Check sheet for the drawn part. Datum: minimum x, y, z corner. Units: mm. Give positions to 0.01 mm unless a question says otherwise; leave off trailing zeros. Write each loop counter-clockwise with the first axis right and the second up, starting at its lowest first coordinate (ties: lowest second). Pieces come first, ordered by that corner, then holes. Notation, with made-up numbers: (26, 60) - (64, 60) arc R25 ccw to (64, 86) - close; hole circle Ø9 at (-27, 9.5). An arc over 180 degrees is marked (long way). Return JSON: item names as keys, results as strings. Group by question number.
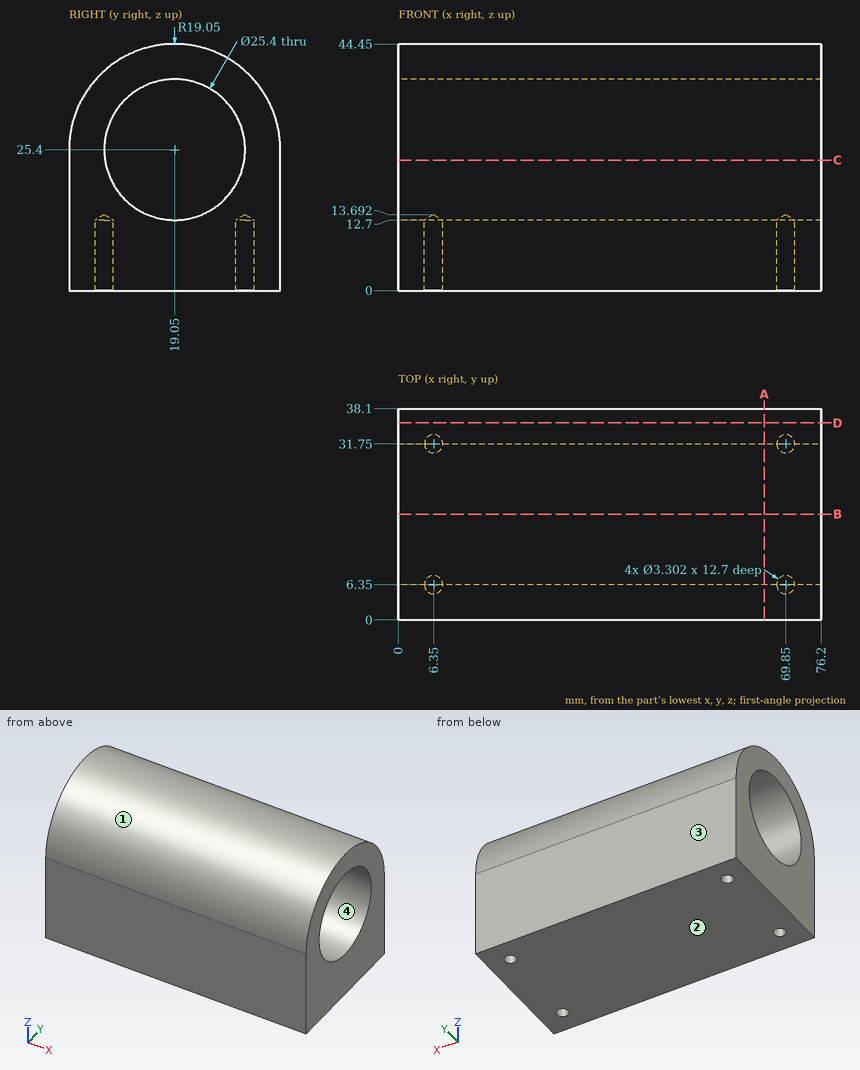
Item 1: Depth check by flat-ended pin: pin 1 (2 mm diameter, centred on x = 6.35, y = 6.35, fed in from +Z); pin 2 (3 mm diameter, centred on x = 6.35, y = 31.75, fed in from -Z); pin 3 (2.5 mm diameter, centred on x = 69.85, y = 6.35, fed in from -Z). Enter the tip coordinate at first touch or a pass-through.
Item 2: Section check B-B on y = 19.05. Record the cut outline in (x, z).
Item 3: Section check C-C on z = 23.5. Record the cut outline in (x, y).
Item 4: Section check A-A on x = 66. Record the cut outline in (y, z).
Item 5: Material ranges on line 1 along Y through (x, z) = (69.85, 7); line 2 along X through (y, z) = (6, 7); line 3 along X through (y, z) = (31, 6), recorded low to high. Write a range as from..to.
Item 6: Mould release check, pull along Z, two halves, no side actions. Record for the marked faces 1, 2, 3 and 4: +Z half, -Z half, draft (parallel to the pull), parting line (faces both ways), or undercut.
Item 7: Section check D-D on y = 35.5. Record the cut outline in (x, z), plus the area to 3 significant figures.
Reply:
{
 "1": {"pin 1": "z = 40.43", "pin 2": "z = 12.79", "pin 3": "z = 12.94"},
 "2": {"outline": "(0, 0) - (76.2, 0) - (76.2, 12.7) - (0, 12.7) - close; (0, 38.1) - (76.2, 38.1) - (76.2, 44.45) - (0, 44.45) - close"},
 "3": {"outline": "(0, 0) - (76.2, 0) - (76.2, 6.49) - (0, 6.49) - close; (0, 31.61) - (76.2, 31.61) - (76.2, 38.1) - (0, 38.1) - close"},
 "4": {"outline": "(0, 0) - (38.1, 0) - (38.1, 25.4) arc R19.05 ccw to (0, 25.4) - close; hole circle Ø25.4 at (19.05, 25.4)"},
 "5": {"line 1": "0..4.7, 8..30.1, 33.4..38.1", "line 2": "0..4.74, 7.96..68.24, 71.46..76.2", "line 3": "0..4.88, 7.82..68.38, 71.32..76.2"},
 "6": {"face 1": "+Z half", "face 2": "-Z half", "face 3": "draft", "face 4": "undercut"},
 "7": {"outline": "(0, 0) - (76.2, 0) - (76.2, 35.01) - (0, 35.01) - close", "area": "2,670 mm²"}
}
